Geometry check sheet. Reference: the model listing, model coordinates, mm. A direction names the side the tool comes from. Round coordinates to 2 decimals unless told otherwise and drop trailing zeros. Loops run counter-clockwise (first coordinate to the right, second up) from the corner with the lowest first, then second, coordinate; pieces in that order, holes last. Notation, with made-up numbers: (-25.5, 61.5) - (-3.5, 61.5) arc R11 ccw to (-3.5, 66.5) - close; hole circle Ø6 at (49.5, -12.75). An arc over 180 degrees is marked (long way). Answer as CSV lines item,"result". Start each with the question number.
1) Cross-section at A-A on y = -2.25. State how many separate pieces and enclosed holes the cut face has, and give its area (3 significant figures).
2) Thickness scan on line 1 along Z through (x, y) = (-50.8, -6.5) (3 decimals); line 2 along X through (y, z) = (-4, -100); line 3 along Z through (x, y) = (7.5, -2.75). Record the ranges inside material, lowest first.
3) Depth check by flat-ended pin: P1, Ø1, axis at y = -11.5, z = -57.5, coming from the -X side; P2, Ø4, axis at y = -6.5, z = -110.5, coming from the -X side; P3, Ø5, axis at y = -7, z = -131.5, coming from the +X side. Enter the tip coordinate at first touch or a pass-through.
4) Cross-section at B-B on x = -60. Record the boundary of the cut face in (y, z), and give its area (3 significant figures).
5) Access from +Z, -Z, +X, -X, +Y, -Y to the whole of each face (thin tool, end or side, straight path). Record for faces 4 (the flat face through (-38.1, -6, -108)), 5 (the flat face through (38.1, -6, -108)), 6 (the cylindrical face through (-0.076, -6.261, -128.587)), 7 (the flat face through (-1, -12.7, -58)).
6) Cross-section at C-C on z = -14. Record the boundary of the cut face in (x, y), and give its area (3 significant figures).
7) Draft check along X on faces 1 (the cylindrical face through (-68.96, -6.26, -68.56)), 2 (the cylindrical face through (-53.97, -6.26, -25.26)), 3 (the flat face through (-1, 0, -58)). Enter one of: released by +X, released by -X, zero draft, split by the parting line, or undercut.
from build123d import *

# Parameters (mm, degrees)
F0_R     = 4.7625
F0_R_2   = 3.175
F1_DEPTH = 12.7


with BuildPart() as f1:
    # F0 (on Front) → F1 (new body)
    with BuildSketch(Plane.XZ):
        with BuildLine():
            Line((50.8, 0), (-50.8, 0))
            ThreePointArc((-50.8, 0), (-68.760512, -7.439488), (-76.2, -25.4))
            Line((-76.2, -25.4), (-76.2, -50.8))
            ThreePointArc((-76.2, -50.8), (-68.760512, -68.760512), (-50.8, -76.2))
            ThreePointArc((-50.8, -76.2), (-41.819744, -79.919744), (-38.1, -88.9))
            Line((-38.1, -88.9), (-38.1, -127))
            ThreePointArc((-38.1, -127), (-30.660512, -144.960512), (-12.7, -152.4))
            Line((-12.7, -152.4), (12.7, -152.4))
            ThreePointArc((12.7, -152.4), (30.660512, -144.960512), (38.1, -127))
            Line((38.1, -127), (38.1, -88.9))
            ThreePointArc((38.1, -88.9), (41.819744, -79.919744), (50.8, -76.2))
            ThreePointArc((50.8, -76.2), (68.760512, -68.760512), (76.2, -50.8))
            Line((76.2, -50.8), (76.2, -25.4))
            ThreePointArc((76.2, -25.4), (68.760512, -7.439488), (50.8, 0))
        make_face()
        with BuildLine():
            ThreePointArc((-7.3025, -137.374798), (-11.016278, -131.75602), (-5.3975, -128.042242))
            ThreePointArc((-5.3975, -128.042242), (0, -128.5875), (5.3975, -128.042242))
            ThreePointArc((5.3975, -128.042242), (11.016278, -131.75602), (7.3025, -137.374798))
            ThreePointArc((7.3025, -137.374798), (0, -138.1125), (-7.3025, -137.374798))
        make_face(mode=Mode.SUBTRACT)
        with Locations((0, -101.6)):
            Circle(F0_R, mode=Mode.SUBTRACT)
        with Locations((-50.8, -25.4)):
            Circle(F0_R_2, mode=Mode.SUBTRACT)
        with Locations((0, -50.8)):
            Circle(F0_R_2, mode=Mode.SUBTRACT)
        with Locations((47.625, -25.4)):
            Circle(F0_R_2, mode=Mode.SUBTRACT)
    extrude(amount=F1_DEPTH)


solid = f1.part
Answer block:
1,separate pieces,"1"
1,enclosed holes,"5"
1,area,"16,300 mm^2"
2,line 1,"z = -76.2 to -28.575, -22.225 to 0"
2,line 2,"x = -38.1 to -4.49, 4.49 to 38.1"
2,line 3,"z = -152.4 to -137.33, -128.09 to 0"
3,P1,"stops at x = -75.43"
3,P2,"stops at x = -38.1"
3,P3,"stops at x = 38.02"
4,outline,"(-12.7, -74.48) - (0, -74.48) - (0, -1.72) - (-12.7, -1.72) - close"
4,area,"924 mm^2"
5,face 4,"-Z, -X, +Y, -Y"
5,face 5,"-Z, +X, +Y, -Y"
5,face 6,"+Y, -Y"
5,face 7,"+Z, -Z, +X, -X, -Y"
6,outline,"(-73.5, -12.7) - (73.5, -12.7) - (73.5, 0) - (-73.5, 0) - close"
6,area,"1,870 mm^2"
7,face 1,"released by -X"
7,face 2,"undercut"
7,face 3,"zero draft"
